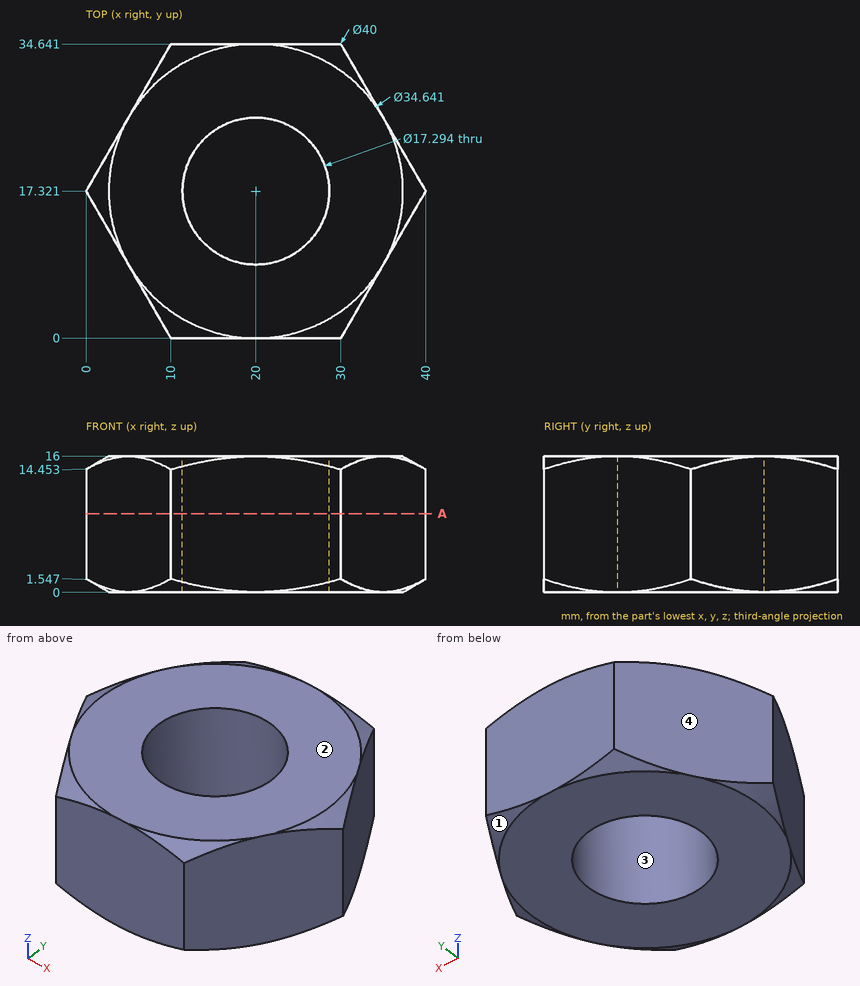
Study the drawing (mm; zero at the part's minimum x, y, z) and answer. Give positions to 0.01 mm unless a question says otherwise; leave off trailing zeros. Write each loop counter-clockwise with the first axis right and the second up, starting at its lowest first coordinate (ties: lowest second). Pieces come first, ordered by that corner, then holes. Notation, with made-up numbers: (56, 46.5) - (104, 46.5) arc R15 cw to (104, 51.5) - close; hole circle Ø9 at (36.25, 46). An arc over 180 degrees is marked (long way). Use CSV: the item, a comma, the result in double quotes. Start each with the question number.
(1) Consider line 1 along X through (y, z) = (10.5, 2.5) (1 decimal); line 2 along X through (y, z) = (21, 13.5) (1 decimal); line 3 along Y through (x, z) = (21, 2.5). Determine where each line is inside the solid, lowest interval first.
(2) Determine the mould class of the marked faces 1, 2, 3 and 4 for opening direction Y: +Y half, -Y half, draft (parallel to the pull), parting line (faces both ways), or undercut.
(3) Find section A-A (z = 9.25). Give the vertices of the cut face in (x, y) (1 decimal).
(4) Given P1, Ø2, axis at y = 25, z = 12.5, coming from the -X side; P2, Ø1, axis at y = 22.5, z = 11.5, coming from the -X side; P3, Ø14, axis at x = 20, y = 17.32, coming from the +Z side; P4, Ø3, axis at y = 5.5, z = 13, coming from the +X side, each flat-ended and moving along its own axis, determine where each tip first touches the part or whether it passes through.
Findings below:
1,line 1,"3.9 to 14.7, 25.3 to 36.1"
1,line 2,"2.1 to 12.2, 27.8 to 37.9"
1,line 3,"0 to 8.73, 25.91 to 34.64"
2,face 1,"parting line"
2,face 2,"draft"
2,face 3,"undercut"
2,face 4,"+Y half"
3,outline,"(0, 17.3) - (10, 0) - (30, 0) - (40, 17.3) - (30, 34.6) - (10, 34.6) - close; hole circle Ø17.3 at (20, 17.3)"
4,P1,"x = 3.86"
4,P2,"x = 2.7"
4,P3,"through"
4,P4,"x = 34.04"
